Autodesk Inventor part; units mm, degrees
ref_plane "РабПлоскость1" through (57, 0, 0) normal (1, 0, 0) x (0, 0, -1)
ref_plane "YZ Plane" through (0, 0, 0) normal (1, 0, 0) x (0, 1, 0)
ref_plane "XZ Plane" through (0, 0, 0) normal (0, 1, 0) x (-1, 0, 0)
sketch "Эскиз1" plane through (0, 0, 0) normal (0, 0, 1) x (1, 0, 0)
  line L0 (0, 0) -> (140, 0)
  line L1 (0, 0) -> (0, 15)
  line L2 (0, 15) -> (12, 15)
  line L3 (12, 15) -> (12, 24)
  line L4 (12, 24) -> (140, 24)
  line L5 (140, 24) -> (140, 0)
  dimension "d1" = 30
  dimension "d2" = 48
  dimension "d3" = 12
  dimension "d4" = 140
revolve "Вращение1" add sketch "Эскиз1" angle 360 about axis through (0, 0, 0) along (1, 0, 0)
ref_plane "РабПлоскость1" through (57, 0, 0) normal (1, 0, 0) x (0, 0, -1)
sketch "Эскиз2" plane through (57, 0, 0) normal (1, 0, 0) x (0, 0, -1)
  arc A0 (0, 40) -> (9.6, 52.8) centre (0, 50) ccw
  circle A1 centre (0, 0) radius 24
  line L0 (-23.04, 6.72) -> (-9.6, 52.8)
  line L1 (0, -43.1124) -> (0, 90.6743)
  line L2 (23.04, 6.72) -> (9.6, 52.8)
  circle A2 centre (0, 50) radius 4
  arc A3 (23.04, 6.72) -> (-23.04, 6.72) centre (0, 0) ccw
  arc A4 (-9.6, 52.8) -> (0, 40) centre (0, 50) ccw
  arc A5 (9.6, 52.8) -> (-9.6, 52.8) centre (0, 50) ccw
  point P0 (0, 0)
  dimension "d7" = 20
  dimension "d8" = 8
  dimension "d13" = 50
extrude "Выдавливание1" add sketch "Эскиз2" against normal blind 8 contours L1 A2 A5 A0 | A0 L2 A1 L1 | A4 A5 L1 A2 | L1 A1 L0 A4
extrude "Выдавливание2" add sketch "Эскиз2" against normal blind 10 contours L1 A2 A5 A0 | A4 A5 L1 A2
mirror "Зеркальное отражение1" about plane through (0, 0, 0) normal (0, 1, 0) of "Выдавливание1", "Выдавливание2"
sketch "Эскиз3" plane through (140, 0, 0) normal (1, 0, 0) x (0, 0, -1)
  circle A0 centre (0, 0) radius 24
hole "Отверстие1" at (140, 0, 0) direction (-1, 0, 0) diameter 36 depth 120
sketch "Эскиз4" plane through (0, 0, 0) normal (-1, 0, 0) x (0, 0, 1)
  line L0 (9, 9) -> (9, -9)
  line L1 (9, -9) -> (-9, -9)
  line L2 (-9, -9) -> (-9, 9)
  line L3 (-9, 9) -> (9, 9)
  point P0 (0, 0)
  point P1 (0, 0)
  dimension "d21" = 18
extrude "Выдавливание3" cut sketch "Эскиз4" against normal up to surface (20 mm away)
thread "Резьба1"
fillet "Сопряжение1" radius 5 1 edges at (12, -24, 0)
chamfer "Фаска1" distance 1 angle 45 1 edges at (140, -24, 0)
properties part number "05.01.003" material "Чугун, серый"
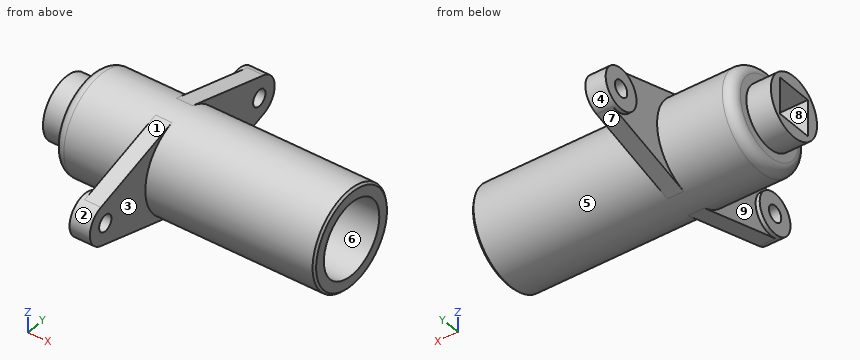
The model under review builds one solid part; all positions refer to its coordinate system, in mm. Face numbers are marked on the shaded views. A direction names the side the tool comes from. Round coordinates to 2 decimals unless told otherwise and drop trailing zeros. Order: outer loops, then holes, each group sorted by start corner. A loop starts at its lowest first (then second) coordinate and runs counter-clockwise, first axis right, second up. Notation, with made-up numbers: M -13,49.25 L 10,49.25 A14 cw 10,58.25 Z; hole C 35,74.25 d3. An arc over 180 degrees is marked long. Use a Markdown table: item, result.
1) Wall thickness on line 1 along Y through (x, z) = (51.5, 0); line 2 along Z through (x, y) = (57.5, 0); line 3 along X through (y, z) = (17, -19): over which ranges is each line inside the solid? List them lowest first. Write a range as [from, to].
Report:
| item | result |
|---|---|
| line 1 | [-60, -54], [-46, -18], [18, 46], [54, 60] |
| line 2 | [-24, -18], [18, 24] |
| line 3 | [49, 57] |
2) Draft analysis for pull direction Y (two halves, no side actions). For the marked faces 1, 2, 3 and 4, state which applies: released by +Y, released by -Y, zero draft, split by the parting line, or undercut.
Report:
| item | result |
|---|---|
| face 1 | released by -Y |
| face 2 | undercut |
| face 3 | zero draft |
| face 4 | undercut |
3) Tool access review of the marked faces 5, 6, 7, 8 and 9: name each direction out of +Z, -Z, +X, -X, +Y, -Y from which nothing blocks a thin tool from reaching the whole face with its end or side.
Report:
| item | result |
|---|---|
| face 5 | none |
| face 6 | +X |
| face 7 | -Z, +X, -X, +Y |
| face 8 | +X, -X |
| face 9 | -X |
4) Consider section C-C (z = 0). Give the number of separate pieces and of enclosed holes in the cut face, then the cut area to 3 significant figures.
Report:
| item | result |
|---|---|
| separate pieces | 4 |
| enclosed holes | 0 |
| area | 2,310 mm^2 |
5) Consider section A-A (y = 0). Write out the cut boundary in (x, z), then the cut area to 3 significant figures.
Report:
| item | result |
|---|---|
| outline | M 0,-15 L 12,-15 L 12,-19 A5 ccw 17,-24 L 139,-24 L 140,-23 L 140,-18 L 20,-18 L 20,-9 L 0,-9 Z; M 0,9 L 20,9 L 20,18 L 140,18 L 140,23 L 139,24 L 17,24 A5 ccw 12,19 L 12,15 L 0,15 Z |
| area | 1,810 mm^2 |
6) Consider section B-B (x = 53). Write out the cut boundary in (y, z), then the cut area to 3 significant figures.
Report:
| item | result |
|---|---|
| outline | M -52.8,-9.6 L -6.72,-23.04 A24 ccw 6.72,-23.04 L 52.8,-9.6 A10 ccw 52.8,9.6 L 6.72,23.04 A24 ccw -6.72,23.04 L -52.8,9.6 A10 ccw Z; hole C -50,0 d8; hole C 0,0 d36; hole C 50,0 d8 |
| area | 2,730 mm^2 |
7) Consider section D-D (y = -42). Write out the cut boundary in (x, z).
Report:
| item | result |
|---|---|
| outline | M 47,-6 L 49,-6 L 49,-12.75 L 57,-12.75 L 57,12.75 L 49,12.75 L 49,6 L 47,6 Z |
8) Insertion check: pin 1 (13 mm diameter, centred on y = -50, z = 0, fed in from -X); pin 2 (6 mm diameter, centred on x = 119, y = 11, fed in from +Z); pin 3 (2 mm diameter, centred on y = -24, z = -6.5, fed in from +X). Each pin has a flat end and moves straight along its axis. Give the tip position at first contact, or say it passes through.
Report:
| item | result |
|---|---|
| pin 1 | x = 47 |
| pin 2 | z = 22.63 |
| pin 3 | x = 139.14 |
